Build history of the part. All positions in model axes, mm. Face numbers are marked on the shaded views. A direction names the side the tool comes from. Round coordinates to 2 decimals unless told otherwise and drop trailing zeros. Write each loop counter-clockwise with the first axis right and the second up, starting at its lowest first coordinate (ties: lowest second). Pieces come first, ordered by that corner, then holes.
from build123d import *

# Parameters (mm, degrees)
F0_W     = 76.2
F0_H     = 32.2935292425
F1_DEPTH = 3.175
F2_R     = 10.16
F3_W     = 18.1224476546
F3_H     = 7.2736367583
F4_DEPTH = 12.7
F5_W     = 101.6
F5_H     = 38.1
F5_W_2   = 18.1224476546
F5_H_2   = 7.2736367583
F6_DEPTH = 25.4
F7_R     = 12.69999
F8_R     = 5.8655823146
F8_R_2   = 2.7147756384
F9_DEPTH = 5.08


# Not quite as in the source:
# - a fillet or chamfer is up to 0.001 mm smaller than in the source, because OpenCascade refuses the exact size


with BuildPart() as f1:
    # F0 (on Top) → F1 (new body)
    with BuildSketch(Plane.XY):
        Rectangle(F0_W, F0_H)
    extrude(amount=F1_DEPTH)

    # F2
    f2_edges = [f1.edges().sort_by_distance(p)[0] for p in [
        (-38.1, -16.146765, 1.5875),
        (38.1, -16.146765, 1.5875),
        (38.1, 16.146765, 1.5875),
        (-38.1, 16.146765, 1.5875),
    ]]
    fillet(f2_edges, radius=F2_R)

    # F3 (on face) → F4 (join)
    with BuildSketch(Plane.XY.offset(3.175)):
        Rectangle(F3_W, F3_H)
    extrude(amount=F4_DEPTH)

    # F5 (on face) → F6 (join)
    with BuildSketch(Plane.XY.offset(15.875)):
        Rectangle(F5_W, F5_H)
        Rectangle(F5_W_2, F5_H_2, mode=Mode.SUBTRACT)
        Rectangle(F5_W_2, F5_H_2)
    extrude(amount=F6_DEPTH)

    # F7 (radius 12.7 in the source; OpenCascade refuses exactly that, so slightly less here)
    f7_edges = [f1.edges().sort_by_distance(p)[0] for p in [
        (-50.8, -19.05, 28.575),
        (0, -19.05, 41.275),
        (0, -19.05, 15.875),
        (50.8, -19.05, 28.575),
        (50.8, 0, 41.275),
        (50.8, 0, 15.875),
        (-50.8, 0, 41.275),
        (-50.8, 0, 15.875),
        (0, 19.05, 15.875),
        (0, 19.05, 41.275),
        (50.8, 19.05, 28.575),
        (-50.8, 19.05, 28.575),
    ]]
    fillet(f7_edges, radius=F7_R)

    # F8 (on face) → F9 (cut)
    with BuildSketch(Plane.XY.offset(41.275)):
        Circle(F8_R)
        with Locations((11.8326274678, 0)):
            Circle(F8_R_2)
    extrude(amount=-F9_DEPTH, mode=Mode.SUBTRACT)


solid = f1.part
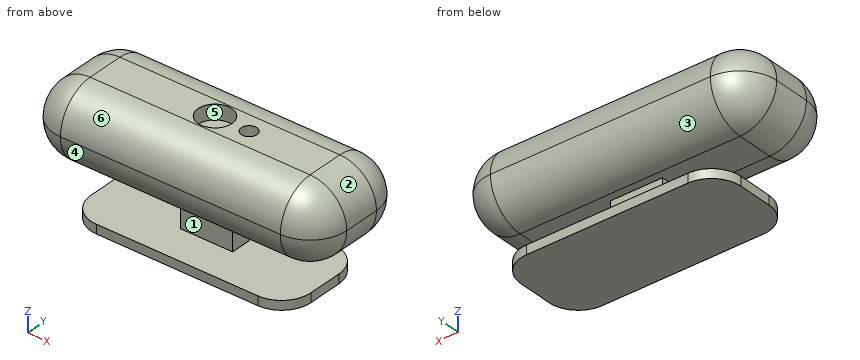
1) Wall check: L1, parallel to Z at x = -10, y = 1 (3 decimals); L2, parallel to Y at x = 0, z = 38.2; L3, parallel to Y at x = 0, z = 39.55. Give the ranges that are in metal, low to high.
Results:
L1: z = 0 to 3.175, 15.875 to 41.275
L2: y = -14.64 to -5.87, 5.87 to 14.64
L3: y = -12.74 to -5.87, 5.87 to 12.74
2) Pin check, flat tips, straight feed: pin 1 Ø9.5 at (x, y) = (0, 0) entering from +Z (3 decimals); pin 2 Ø1.6 at (x, z) = (-12.5, 1) entering from -Y; pin 3 Ø1.5 at (y, z) = (-6.5, 20.5) entering from -X. Stop position of each tip, or through.
Results:
pin 1: stops at z = 36.195
pin 2: stops at y = -16.15
pin 3: stops at x = -48.47
3) Which spindle directions (+Z, -Z, +X, -X, +Y, -Y) get a long thin tool onto all of the face, cutting with end or side? Do the marked faces 1, 2 and 3. Say none if no direction does.
Results:
face 1: +X, -X, -Y
face 2: +Z, +X, +Y, -Y
face 3: +X, -X, +Y
4) Slice it at D-D (z = 27). Write the cut outline in (x, y), plus the area to 3 significant figures.
Results:
outline: (-50.7, -6.35) arc R12.6 ccw to (-38.1, -18.95) - (38.1, -18.95) arc R12.6 ccw to (50.7, -6.35) - (50.7, 6.35) arc R12.6 ccw to (38.1, 18.95) - (-38.1, 18.95) arc R12.6 ccw to (-50.7, 6.35) - close
area: 3,710 mm2
5) Mould opens along Z. For the marked faces 4, 5 and 6 say: released by +Z, released by -Z, zero draft, split by the parting line, or undercut.
Results:
face 4: undercut
face 5: zero draft
face 6: released by +Z
